Geometry check sheet. Reference: the model listing, model coordinates, mm. Face numbers are marked on the shaded views. A direction names the side the tool comes from. Coordinates: 2 decimals unless noted, no trailing zeros. Order: outer loops, then holes, each group sorted by start corner. A loop starts at its lowest first (then second) coordinate and runs counter-clockwise, first axis right, second up. Notation, with made-up numbers: (-35.5, 14) - (-3.5, 14) arc R25 cw to (-3.5, 26) - close; hole circle Ø9 at (52.25, 17.25). An arc over 180 degrees is marked (long way). Put each result on its own line as item: value.
from build123d import *

# Parameters (mm, degrees)
SKETCH1_W           = 203.2
SKETCH1_H           = 25.4
BOSS_EXTRUDE1_DEPTH = 101.6
SKETCH2_W           = 25.4
SKETCH2_H           = 6.35
CUT_EXTRUDE1_DEPTH  = 229.6
BOSS_EXTRUDE2_REACH = 235.091
SKETCH4_R           = 19.05
SKETCH4_R_2         = 9.525
BOSS_EXTRUDE3_DEPTH = 12.7
BOSS_EXTRUDE4_DEPTH = 101.6
BOSS_EXTRUDE5_DEPTH = 22.225
SKETCH7_R           = 25.4
SKETCH7_R_2         = 12.7
CUT_EXTRUDE4_DEPTH  = 12.7
CUT_EXTRUDE5_REACH  = 277.657
SKETCH8_R           = 12.7
CUT_EXTRUDE6_DEPTH  = 6.35


with BuildPart() as part:
    # Sketch1 → Boss-Extrude1 (new body)
    with BuildSketch(Plane.XY):
        with Locations((-101.6, 12.7)):
            Rectangle(SKETCH1_W, SKETCH1_H)
    extrude(amount=-BOSS_EXTRUDE1_DEPTH)

    # Sketch2 → Cut-Extrude1 (cut, through all)
    with BuildSketch(Plane.XY):
        with Locations((-139.7, 22.225)):
            Rectangle(SKETCH2_W, SKETCH2_H)
    extrude(amount=-CUT_EXTRUDE1_DEPTH, mode=Mode.SUBTRACT)

    # Sketch3 → Boss-Extrude2 (add, up to next)
    with BuildSketch(Plane(origin=(0, 19.05, 10.998522628), x_dir=(-1, 0, 0), z_dir=(0, 0.866025403784438, 0.500000000000001)), mode=Mode.PRIVATE) as boss_extrude2_sk1:
        with BuildLine():
            Line((38.1, -12.7), (38.1, -57.15))
            ThreePointArc((38.1, -57.15), (69.85, -88.9), (101.6, -57.15))
            Line((101.6, -57.15), (101.6, -12.7))
            Line((101.6, -12.7), (38.1, -12.7))
        make_face()
    boss_extrude2_tool1 = extrude(boss_extrude2_sk1.sketch, amount=-BOSS_EXTRUDE2_REACH, mode=Mode.PRIVATE) - part.part
    add(boss_extrude2_tool1.solids().sort_by_distance((-69.85, 42.927534, -30.35858))[0])

    # Sketch4 → Boss-Extrude3 (add)
    with BuildSketch(Plane(origin=(0, 19.05, 10.998522628), x_dir=(1, 0, 0), z_dir=(0, 0.8660254037844382, 0.5000000000000011))):
        with Locations(Location((-69.85, 57.15, 0), (0, 0, 270))):
            Circle(SKETCH4_R)
        with Locations(Location((-69.85, 57.15, 0), (0, 0, 270))):
            Circle(SKETCH4_R_2, mode=Mode.SUBTRACT)
    extrude(amount=BOSS_EXTRUDE3_DEPTH)

    # Sketch5 → Boss-Extrude4 (add)
    with BuildSketch(Plane.XY):
        Polygon((-203.2, 0), (-283.328628158, 114.435540587), (-262.522166233, 129.00438207), (-182.393538075, 14.568841483), align=None)
    extrude(amount=-BOSS_EXTRUDE4_DEPTH)

    # Sketch6 → Boss-Extrude5 (add)
    with BuildSketch(Plane(origin=(-146.979381596, 209.908310859, 0), x_dir=(0.8191520442889892, 0.5735764363510499, 0), z_dir=(-0.5735764363510498, 0.8191520442889891, 0))):
        with BuildLine():
            Line((-166.4516954, 0), (-102.9516954, 0))
            ThreePointArc((-102.9516954, 0), (-52.1516954, 50.8), (-102.9516954, 101.6))
            Line((-102.9516954, 101.6), (-166.4516954, 101.6))
            Line((-166.4516954, 101.6), (-166.4516954, 0))
        make_face()
    extrude(amount=-BOSS_EXTRUDE5_DEPTH)

    # Sketch7 → Cut-Extrude4 (cut)
    with BuildSketch(Plane(origin=(-146.979381596, 209.908310859, 0), x_dir=(0.8191520442889892, 0.5735764363510499, 0), z_dir=(-0.5735764363510498, 0.8191520442889891, 0))):
        with Locations(Location((-102.9516954, 50.8, 0), (0, 0, 180))):
            Circle(SKETCH7_R)
        with Locations(Location((-102.9516954, 50.8, 0), (0, 0, 180))):
            Circle(SKETCH7_R_2, mode=Mode.SUBTRACT)
    extrude(amount=-CUT_EXTRUDE4_DEPTH, mode=Mode.SUBTRACT)

    # Sketch8 → Cut-Extrude5 (cut, up to next)
    with BuildSketch(Plane(origin=(-146.979381596, 209.908310859, 0), x_dir=(0.8191520442889892, 0.5735764363510499, 0), z_dir=(-0.5735764363510498, 0.8191520442889891, 0)), mode=Mode.PRIVATE) as cut_extrude5_sk1:
        with Locations(Location((-102.9516954, 50.8, 0), (0, 0, 180))):
            Circle(SKETCH8_R)
    cut_extrude5_tool1 = extrude(cut_extrude5_sk1.sketch, amount=-CUT_EXTRUDE5_REACH, mode=Mode.PRIVATE) & part.part
    add(cut_extrude5_tool1.solids().sort_by_distance((-231.312473, 150.857644, -50.8))[0], mode=Mode.SUBTRACT)

    # Sketch9 → Cut-Extrude6 (cut)
    with BuildSketch(Plane(origin=(-146.979381596, 209.908310859, 0), x_dir=(0.8191520442889892, 0.5735764363510499, 0), z_dir=(-0.5735764363510498, 0.8191520442889891, 0))):
        with BuildLine():
            ThreePointArc((-54.695873212, 34.925), (-52.1516954, 50.8), (-54.695873212, 66.675))
            Line((-54.695873212, 66.675), (-83.123826755, 66.675))
            ThreePointArc((-83.123826755, 66.675), (-78.985178511, 59.212257022), (-77.5516954, 50.8))
            ThreePointArc((-77.5516954, 50.8), (-78.985178511, 42.387742978), (-83.123826755, 34.925))
            Line((-83.123826755, 34.925), (-54.695873212, 34.925))
        make_face()
        with BuildLine():
            ThreePointArc((-122.779564044, 34.925), (-128.3516954, 50.8), (-122.779564044, 66.675))
            Line((-122.779564044, 66.675), (-166.4516954, 66.675))
            Line((-166.4516954, 66.675), (-166.4516954, 34.925))
            Line((-166.4516954, 34.925), (-122.779564044, 34.925))
        make_face()
    extrude(amount=-CUT_EXTRUDE6_DEPTH, mode=Mode.SUBTRACT)


solid = part.part
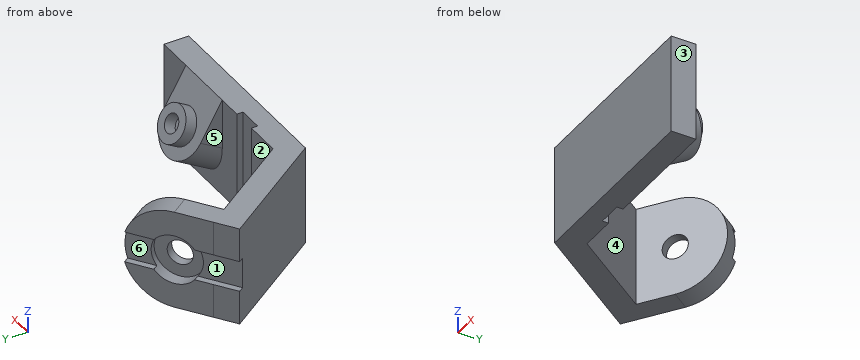
Q1. Section check C-C on z = -41.5. State how many separate pieces and enclosed holes the cut face has, then the cut area to 3 significant figures.
Answer block:
separate pieces: 2
enclosed holes: 1
area: 10,900 mm^2
Q2. Section check A-A on x = -54. Record the boundary of the cut face in (y, z).
Answer block:
outline: (0, -101.6) - (25.4, -101.6) - (25.4, -83.09) - (61.38, -62.32) - (52.91, -47.65) - (63.91, -41.3) - (53.34, -22.99) - (42.34, -29.34) - (25.4, 0) - (0, 0) - close
Q3. Section check D-D on y = 100.5. Record the boundary of the cut face in (x, z).
Answer block:
outline: (-273.57, -101.6) - (-242.56, -101.6) - (-242.56, 0) - (-273.57, 0) - close
Q4. Thickness scan on L1, parallel to Y at x = -132.5, z = -85; L2, parallel to Y at x = -165, z = -96; L3, parallel to X at y = 19.5, z = -32. Record the ranges inside material, lowest first. Write a range as [from, to].
Answer block:
L1: y = [0, 19.05]
L2: y = [0, 25.4]
L3: x = [-216.85, -152.4], [-127, 0]
Q5. Section check B-B on z = -96. Record the boundary of the cut face in (x, y).
Answer block:
outline: (-283.33, 114.44) - (-203.2, 0) - (0, 0) - (0, 25.4) - (-127, 25.4) - (-127, 19.05) - (-152.4, 19.05) - (-152.4, 25.4) - (-189.98, 25.4) - (-249.77, 110.8) - (-199.57, 145.95) - (-212.32, 164.16) - close
Q6. Depth check by flat-ended pin: pin 1 Ø10 at (x, z) = (-75.5, -69.5) entering from +Y; pin 2 Ø8 at (x, z) = (-166, -24.5) entering from +Y; pin 3 Ø12 at (y, z) = (148, -34.5) entering from +X. Enter the tip coordinate at first touch or a pass-through.
Answer block:
pin 1: stops at y = 63.46
pin 2: stops at y = 25.4
pin 3: stops at x = -188.08
Q7. Access from +Z, -Z, +X, -X, +Y, -Y to the whole of each face (thin tool, end or side, straight path). Record for the marked faces 4, 5 and 6.
Answer block:
face 4: +Z, -Z
face 5: +Z, -Z, +Y
face 6: -X, +Y
Q8. Draft check along X on the marked faces 1, 2 and 3. Enter one of: pulls with the +X half, pulls with the -X half, needs draft (parallel to the pull), parting line crosses it, or undercut.
Answer block:
face 1: pulls with the -X half
face 2: undercut
face 3: pulls with the +X half
